Can you work these out from the drawing? Everything is in mm from the part's minimum corner. A direction names the side the tool comes from. Give positions to 0.01 mm unless a question says otherwise; leave off trailing zeros. Write each loop counter-clockwise with the first axis right and the second up, starting at its lowest first coordinate (ties: lowest second). Pieces come first, ordered by that corner, then holes. Notation, with made-up numbers: (-4.5, -34) - (52.5, -34) arc R7 cw to (52.5, -23) - close; hole circle Ø2 at (31, 30.25). An arc over 180 degrees is marked (long way). Use a Markdown table: item, result.
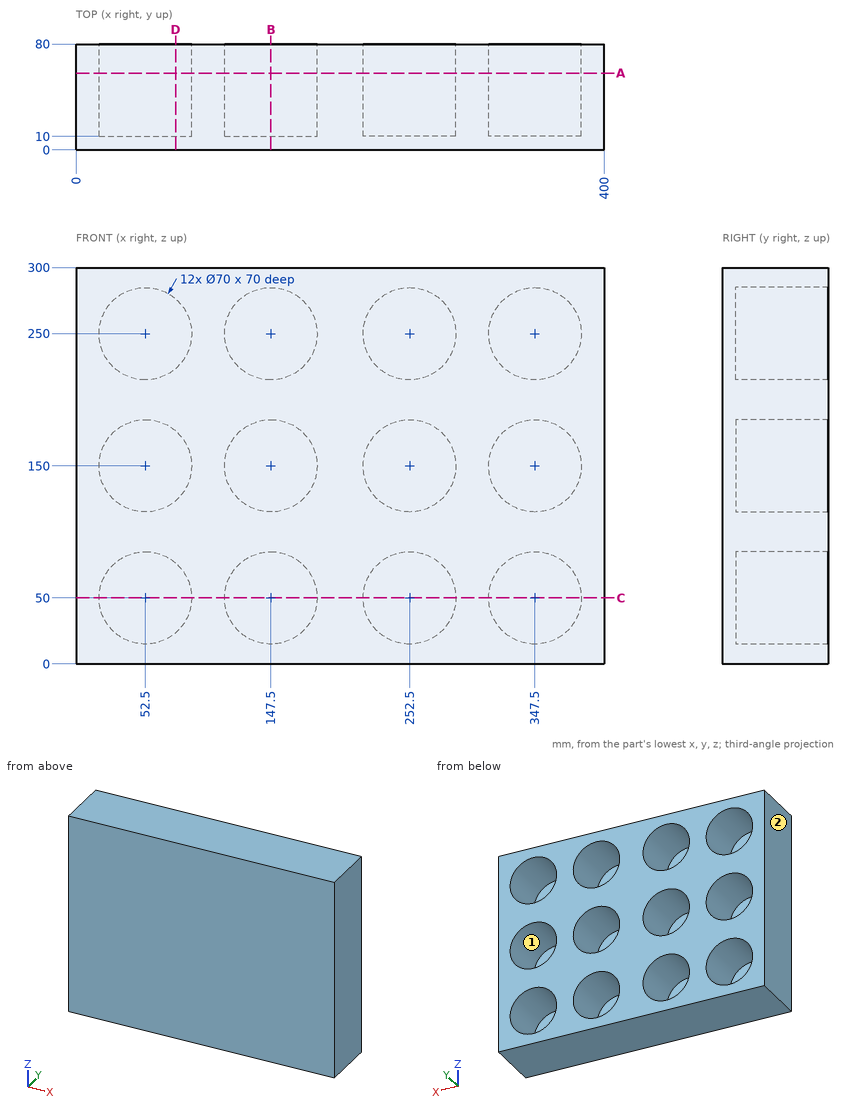
Item 1: If we section it at B-B, the plane x = 147.5: Write out the boundary of the cut face in (y, z).
Values:
| item | result |
|---|---|
| outline | (0, 0) - (80, 0) - (80, 15) - (10, 15) - (10, 85) - (80, 85) - (80, 115) - (10, 115) - (10, 185) - (80, 185) - (80, 215) - (10, 215) - (10, 285) - (80, 285) - (80, 300) - (0, 300) - close |
Item 2: If we section it at A-A, the plane y = 58: Count the separate pieces of the cut face and the enclosed holes in it, plus the area to 3 significant figures.
Values:
| item | result |
|---|---|
| separate pieces | 1 |
| enclosed holes | 12 |
| area | 73,800 mm2 |
Item 3: I need wall thicknesses on line 1 along Z through (x, y) = (347, 50); line 2 along Z through (x, y) = (55, 20); line 3 along X through (y, z) = (29, 150). Which ranges of each line are inside material? Lowest first, please. Write a range as [from, to].
Values:
| item | result |
|---|---|
| line 1 | z = [0, 15], [85, 115], [185, 215], [285, 300] |
| line 2 | z = [0, 15.09], [84.91, 115.09], [184.91, 215.09], [284.91, 300] |
| line 3 | x = [0, 17.5], [87.5, 112.5], [182.5, 217.5], [287.5, 312.5], [382.5, 400] |
Item 4: For the marked faces 1 and 2, which set-ups out of +Z, -Z, +X, -X, +Y, -Y let a thin tool reach every point of the face, with its end or its side?
Values:
| item | result |
|---|---|
| face 1 | +Y |
| face 2 | +Z, -Z, -X, +Y, -Y |
Item 5: Will this pin go through, and if not, where does the flat tip stop? pin 1 Ø10 at (x, z) = (346, 213.5) entering from -Y.
Values:
| item | result |
|---|---|
| pin 1 | stops at y = 0 |
Item 6: If we section it at C-C, the plane z = 50: Write out the boundary of the cut face in (x, y).
Values:
| item | result |
|---|---|
| outline | (0, 0) - (400, 0) - (400, 80) - (382.5, 80) - (382.5, 10) - (312.5, 10) - (312.5, 80) - (287.5, 80) - (287.5, 10) - (217.5, 10) - (217.5, 80) - (182.5, 80) - (182.5, 10) - (112.5, 10) - (112.5, 80) - (87.5, 80) - (87.5, 10) - (17.5, 10) - (17.5, 80) - (0, 80) - close |
Item 7: If we section it at D-D, the plane x = 75.5: Write out the boundary of the cut face in (y, z), plus the area to 3 significant figures.
Values:
| item | result |
|---|---|
| outline | (0, 0) - (80, 0) - (80, 23.62) - (10, 23.62) - (10, 76.38) - (80, 76.38) - (80, 123.62) - (10, 123.62) - (10, 176.38) - (80, 176.38) - (80, 223.62) - (10, 223.62) - (10, 276.38) - (80, 276.38) - (80, 300) - (0, 300) - close |
| area | 12,900 mm2 |
